```python
from build123d import *

# Parameters (mm, degrees)
F1_DEPTH      = 50.8
F2_W          = 31.75
F2_H          = 35.56
F2_W_2        = 25.4
F3_DEPTH      = 38.1
F4_W          = 31.75
F4_H          = 35.56
F4_W_2        = 25.4
F5_DEPTH      = 38.1
F6_R          = 4.445
F7_DEPTH      = 43.181
F7_DEPTH_BACK = 5.08
F8_W          = 38.1
F8_H          = 72.0014913142
F8_H_2        = 84.6492543429
F9_DEPTH      = 48.26
F10_R         = 25.4
F11_W         = 133.5816735625
F11_H         = 43.6864450194
F12_DEPTH     = 176.022


with BuildPart() as f1:
    # F0 (on Top) → F1 (new body)
    with BuildSketch(Plane.XY):
        with BuildLine():
            Line((63.5, 74.1007456571), (18.0570790654, 74.1007456571))
            ThreePointArc((18.0570790654, 74.1007456571), (0, 69.1302912268), (-18.0570790654, 74.1007456571))
            Line((-18.0570790654, 74.1007456571), (-63.5, 74.1007456571))
            Line((-63.5, 74.1007456571), (-63.5, 0))
            Line((-63.5, 0), (63.5, 0))
            Line((63.5, 0), (63.5, 74.1007456571))
        make_face()
        with BuildLine():
            Line((63.5, -74.1007456571), (63.5, 0))
            Line((63.5, 0), (-63.5, 0))
            Line((-63.5, 0), (-63.5, -74.1007456571))
            Line((-63.5, -74.1007456571), (-18.0570790654, -74.1007456571))
            ThreePointArc((-18.0570790654, -74.1007456571), (0, -69.1302912268), (18.0570790654, -74.1007456571))
            Line((18.0570790654, -74.1007456571), (63.5, -74.1007456571))
        make_face()
        with BuildLine():
            ThreePointArc((35.2848543866, -104.4151456134), (30.6770464236, -86.9812770867), (18.0570790654, -74.1007456571))
            ThreePointArc((18.0570790654, -74.1007456571), (0, -69.1302912268), (-18.0570790654, -74.1007456571))
            ThreePointArc((-18.0570790654, -74.1007456571), (-30.6770464236, -86.9812770867), (-35.2848543866, -104.4151456134))
            ThreePointArc((-35.2848543866, -104.4151456134), (0, -139.7), (35.2848543866, -104.4151456134))
        make_face()
        with BuildLine():
            Line((-18.0570790654, -74.1007456571), (-63.5, -74.1007456571))
            Line((-63.5, -74.1007456571), (-35.2848543866, -104.4151456134))
            ThreePointArc((-35.2848543866, -104.4151456134), (-30.6770464236, -86.9812770867), (-18.0570790654, -74.1007456571))
        make_face()
        with BuildLine():
            Line((35.2848543866, -104.4151456134), (63.5, -74.1007456571))
            Line((63.5, -74.1007456571), (18.0570790654, -74.1007456571))
            ThreePointArc((18.0570790654, -74.1007456571), (30.6770464236, -86.9812770867), (35.2848543866, -104.4151456134))
        make_face()
        with BuildLine():
            ThreePointArc((18.0570790654, 74.1007456571), (30.6770464236, 86.9812770867), (35.2848543866, 104.4151456134))
            ThreePointArc((35.2848543866, 104.4151456134), (0, 139.7), (-35.2848543866, 104.4151456134))
            ThreePointArc((-35.2848543866, 104.4151456134), (-30.6770464236, 86.9812770867), (-18.0570790654, 74.1007456571))
            ThreePointArc((-18.0570790654, 74.1007456571), (0, 69.1302912268), (18.0570790654, 74.1007456571))
        make_face()
        with BuildLine():
            Line((63.5, 74.1007456571), (35.2848543866, 104.4151456134))
            ThreePointArc((35.2848543866, 104.4151456134), (30.6770464236, 86.9812770867), (18.0570790654, 74.1007456571))
            Line((18.0570790654, 74.1007456571), (63.5, 74.1007456571))
        make_face()
        with BuildLine():
            ThreePointArc((-18.0570790654, 74.1007456571), (-30.6770464236, 86.9812770867), (-35.2848543866, 104.4151456134))
            Line((-35.2848543866, 104.4151456134), (-63.5, 74.1007456571))
            Line((-63.5, 74.1007456571), (-18.0570790654, 74.1007456571))
        make_face()
    extrude(amount=F1_DEPTH)

    # F2 (on face) → F3 (cut)
    with BuildSketch(Plane.YZ.offset(63.5)):
        with Locations((-58.2257456571, 25.4)):
            Rectangle(F2_W, F2_H)
        with Locations((-86.8007456571, 25.4)):
            Rectangle(F2_W_2, F2_H)
        with Locations((86.8007456571, 25.4)):
            Rectangle(F2_W_2, F2_H)
        with Locations((58.2257456571, 25.4)):
            Rectangle(F2_W, F2_H)
    extrude(amount=-F3_DEPTH, mode=Mode.SUBTRACT)

    # F4 (on face) → F5 (cut)
    with BuildSketch(Plane(origin=(-63.5, 0, 0), x_dir=(0, -1, 0), z_dir=(-1, 0, 0))):
        with Locations((-58.2257456571, 25.4)):
            Rectangle(F4_W, F4_H)
        with Locations((-86.8007456571, 25.4)):
            Rectangle(F4_W_2, F4_H)
        with Locations((58.2257456571, 25.4)):
            Rectangle(F4_W, F4_H)
        with Locations((86.8007456571, 25.4)):
            Rectangle(F4_W_2, F4_H)
    extrude(amount=-F5_DEPTH, mode=Mode.SUBTRACT)

    # F6 (on face) → F7 (cut, two sides)
    with BuildSketch(Plane.XY.offset(7.62)) as f7_sk:
        with Locations((-44.45, 70.9257456571)):
            Circle(F6_R)
        with Locations((-44.45, -70.9257456571)):
            Circle(F6_R)
        with Locations((44.45, 70.9257456571)):
            Circle(F6_R)
        with Locations((44.45, -70.9257456571)):
            Circle(F6_R)
    extrude(amount=F7_DEPTH, mode=Mode.SUBTRACT)
    extrude(f7_sk.sketch, amount=-F7_DEPTH_BACK, mode=Mode.SUBTRACT)

    # F8 (on face) → F9 (cut)
    with BuildSketch(Plane.XY.offset(50.8)):
        Rectangle(F8_W, F8_H)
        with Locations((38.1, 0)):
            Rectangle(F8_W, F8_H)
        with Locations((0, -78.3253728285)):
            Rectangle(F8_W, F8_H_2)
        with Locations((0, 78.3253728285)):
            Rectangle(F8_W, F8_H_2)
        with Locations((-38.1, 0)):
            Rectangle(F8_W, F8_H)
    extrude(amount=-F9_DEPTH, mode=Mode.SUBTRACT)

    # F10
    f10_edges = [f1.edges().sort_by_distance(p)[0] for p in [
        (-25.4, 42.350746, 25.4),
        (-25.4, -42.350746, 25.4),
        (25.4, -42.350746, 25.4),
        (25.4, 42.350746, 25.4),
        (19.05, -36.000746, 26.67),
        (-19.05, -36.000746, 26.67),
        (19.05, 36.000746, 26.67),
        (-19.05, 36.000746, 26.67),
    ]]
    fillet(f10_edges, radius=F10_R)

    # F11 (on Front) → F12 (cut, symmetric)
    with BuildSketch(Plane.XZ):
        with Locations((3.2908367813, 28.9567774903)):
            Rectangle(F11_W, F11_H)
    extrude(amount=F12_DEPTH, both=True, mode=Mode.SUBTRACT)


solid = f1.part
```
Model file for the job. Use its own axes, mm. A direction names the side the tool comes from. Coordinates: 2 decimals unless noted, no trailing zeros. Write each loop counter-clockwise with the first axis right and the second up, starting at its lowest first coordinate (ties: lowest second). Pieces come first, ordered by that corner, then holes. Notation, with made-up numbers: (-15, 88.25) - (11, 88.25) arc R9 cw to (11, 100.25) - close; hole circle Ø11 at (59, 14.5). An arc over 180 degrees is marked (long way). One line per item, written item: value. Start each with the question number.
1. Tool access for faces 1 (the cylindrical face through (41.174, -67.922, 4.859)), 2 (the flat face through (-1, 2, 0)): list every direction of +Z, -Z, +X, -X, +Y, -Y with a clear straight run to the whole face (end or side of a thin tool).
2. Slice it at B-B (y = -87). Write the cut outline in (x, z), plus the area to 3 significant figures.
3. Flat gauge pins, fed straight in: pin 1 (4.5 mm diameter, centred on x = -44, y = 70, fed in from +Z); pin 2 (2.5 mm diameter, centred on x = 2.5, z = 4.5, fed in from -Y); pin 3 (2.5 mm diameter, centred on x = 49.5, z = 6, fed in from -Y). Where does each tip first touch, or does it go through?
4. Probe line 1 (X direction, y = -20.5, z = 3.5); line 2 (X direction, y = 68, z = 3.25); line 3 (Y direction, x = 40.5, z = 3). List the from-to ranges inside material, lowest first. Write a range as from..to.
5. Slice it at C-C (z = 5.25). Write the cut outline in (x, y) (3 decimals).
6. Slice it at A-A (x = 0). Write the cut outline in (y, z).
7. Mould opens along Y. For faces 3 (the flat face through (-49.195, 89.47, 3.507)), 4 (the cylindrical face through (41.174, 73.93, 4.859)), 5 (the flat face through (63.5, -1, 4)), 6 (the flat face through (-1, 2, 2.54)) say: released by +Y, released by -Y, zero draft, split by the parting line, or undercut.
Answers below:
1. face 1: +Z
1. face 2: -Z, +X, -X, +Y, -Y
2. outline: (-51.49, 0) - (51.49, 0) - (51.49, 7.11) - (19.05, 7.11) - (19.05, 2.54) - (-19.05, 2.54) - (-19.05, 7.11) - (-51.49, 7.11) - close
2. area: 558 mm^2
3. pin 1: stops at z = 2.54
3. pin 2: stops at y = -139.68
3. pin 3: stops at y = -90.49
4. line 1: x = -63.5..-57.15, 57.15..63.5
4. line 2: x = -63.5..-47.8, -41.1..-19.05, 19.05..41.1, 47.8..63.5
4. line 3: y = -98.81..-72.96, -68.89..-36.31, 36.31..68.89, 72.96..98.81
5. outline: (-63.5, -74.101) - (-35.285, -104.415) arc R35.285 ccw to (35.285, -104.415) - (63.5, -74.101) - (63.5, 74.101) - (35.285, 104.415) arc R35.285 ccw to (-35.285, 104.415) - (-63.5, 74.101) - close; hole (-57.15, -36.001) - (-44.45, -36.001) arc R25.4 cw to (-19.05, -61.401) - (-19.05, -120.65) - (19.05, -120.65) - (19.05, -61.401) arc R25.4 cw to (44.45, -36.001) - (57.15, -36.001) - (57.15, 36.001) - (44.45, 36.001) arc R25.4 cw to (19.05, 61.401) - (19.05, 120.65) - (-19.05, 120.65) - (-19.05, 61.401) arc R25.4 cw to (-44.45, 36.001) - (-57.15, 36.001) - close; hole circle Ø8.89 at (-44.45, -70.926); hole circle Ø8.89 at (-44.45, 70.926); hole circle Ø8.89 at (44.45, -70.926); hole circle Ø8.89 at (44.45, 70.926)
6. outline: (-139.7, 0) - (139.7, 0) - (139.7, 7.11) - (120.65, 7.11) - (120.65, 2.54) - (-120.65, 2.54) - (-120.65, 7.11) - (-139.7, 7.11) - close
7. face 3: released by +Y
7. face 4: undercut
7. face 5: zero draft
7. face 6: undercut
